Source: CAD feature listing. Evaluate the final solid. Frame: model axes, mm. A direction names the side the tool comes from. Coordinates: 2 decimals unless noted, no trailing zeros. Write each loop counter-clockwise with the first axis right and the second up, starting at its lowest first coordinate (ties: lowest second). Pieces come first, ordered by that corner, then holes. Notation, with made-up numbers: (-16.75, 61.25) - (15.25, 61.25) arc R14 cw to (15.25, 68.25) - close; hole circle Ø6 at (14, 13.25). An arc over 180 degrees is marked (long way). One line per question, with ' | ' between items. Start each with the question number.
Q1. Access query for faces 1 (the face through (216.99, 45.35, -92.85)), 2 (the face through (110, 25, -100)), 3 (the face through (171, 23, -91)), 4 (the face through (12.72, 11.89, -33.46)). Directions: +Z, -Z, +X, -X, +Y, -Y. A direction counts if a zero-diameter tool reaches every point of the face in a straight line with its end or side. Return the directions, or none.
Q2. Cut plane D-D, the plane z = -15. Return loops of the section in (x, y), plus the area to 3 significant figures.
Q3. Cut plane A-A, the plane y = 51.5. Give the number of separate pieces and of enclosed holes in the cut face, plus the area to 3 significant figures.
Q4. Cut plane C-C, the plane y = 12.5. Return loops of the section in (x, z).
Q5. Draft query along X for faces 5 (the face through (18, 5, -45)), 6 (the face through (108, 20, -51)), 7 (the face through (220, 9, -55)). Return one class per face: +X half, -X half, draft (parallel to the pull), parting line (faces both ways), or undercut.
Q6. Cut plane B-B, the plane x = 110. Return loops of the section in (y, z).
Q7. Line query: line 1 (X direction, y = 16, z = -44.5); line 2 (Z direction, x = 202, y = 8); line 3 (X direction, y = 11.25, z = -15). Output: solid intervals per line, ascending.
Q8. Contact query for flat-ended pins moving along their axis: P1, Ø4.5, axis at x = 43.5, z = -106, coming from the +Y side; P2, Ø10, axis at x = 111, z = -37, coming from the -Y side; P3, Ø18.5, axis at x = 107.5, z = -15.5, coming from the +Y side; P4, Ø25, axis at x = 72, y = 55, coming from the +Z side. Output: stop coordinate, or through.
```python
from build123d import *

# Parameters (mm, degrees)
SKETCH1_W           = 220
SKETCH1_H           = 110
BOSS_EXTRUDE1_DEPTH = 20
SKETCH2_R           = 12.49
SKETCH2_R_2         = 7.6
CUT_EXTRUDE1_DEPTH  = 15
SKETCH3_W           = 220
SKETCH3_H           = 20
BOSS_EXTRUDE2_DEPTH = 50
CHAMFER1_SIZE       = 1
FILLET1_R           = 1
FILLET2_R           = 10
SKETCH4_R           = 11.5
CUT_EXTRUDE2_DEPTH  = 5
SKETCH5_W           = 46.94076836
SKETCH5_H           = 60
SKETCH5_W_2         = 45
SKETCH5_H_2         = 90
CUT_EXTRUDE3_DEPTH  = 256.734237051
FILLET4_R           = 5
SKETCH6_R           = 3.2
CUT_EXTRUDE4_DEPTH  = 10


with BuildPart() as part:
    # Sketch1 → Boss-Extrude1 (new body)
    with BuildSketch(Plane(origin=(0, 0, 0), x_dir=(1, 0, 0), z_dir=(0, 1, 0))):
        with Locations((110, 55)):
            Rectangle(SKETCH1_W, SKETCH1_H)
    extrude(amount=BOSS_EXTRUDE1_DEPTH)

    # Sketch2 → Cut-Extrude1 (cut)
    with BuildSketch(Plane(origin=(0, 20, 0), x_dir=(1, 0, 0), z_dir=(0, 1, 0))):
        with Locations(Location((17.5, 45, 0), (0, 0, 270))):
            Circle(SKETCH2_R)
        with Locations(Location((202.5, 45, 0), (0, 0, 90))):
            Circle(SKETCH2_R)
        with Locations(Location((110, 15, 0), (0, 0, 270))):
            Circle(SKETCH2_R_2)
    extrude(amount=-CUT_EXTRUDE1_DEPTH, mode=Mode.SUBTRACT)

    # Sketch3 → Boss-Extrude2 (add)
    with BuildSketch(Plane(origin=(0, 20, 0), x_dir=(1, 0, 0), z_dir=(0, 1, 0))):
        with Locations((110, 100)):
            Rectangle(SKETCH3_W, SKETCH3_H)
    extrude(amount=BOSS_EXTRUDE2_DEPTH)

    # Chamfer1
    chamfer1_edges = [part.edges().sort_by_distance(p)[0] for p in [
        (17.5, 20, -57.49),
        (202.5, 20, -32.51),
    ]]
    chamfer(chamfer1_edges, length=CHAMFER1_SIZE)

    # Fillet1
    fillet1_edges = [part.edges().sort_by_distance(p)[0] for p in [
        (202.5, 19, -32.51),
        (17.5, 19, -57.49),
    ]]
    fillet(fillet1_edges, radius=FILLET1_R)

    # Fillet2
    fillet2_edges = [part.edges().sort_by_distance(p)[0] for p in [
        (220, 45, -90),
        (0, 45, -90),
        (0, 35, -110),
        (0, 10, 0),
        (220, 35, -110),
        (220, 10, 0),
    ]]
    fillet(fillet2_edges, radius=FILLET2_R - 0.0001)  # a hair under: the kernel refuses the full size

    # Sketch4 → Cut-Extrude2 (cut)
    with BuildSketch(Plane(origin=(0, 20, 0), x_dir=(1, 0, 0), z_dir=(0, 1, 0))):
        with Locations(Location((110, 15, 0), (0, 0, 270))):
            Circle(SKETCH4_R)
    extrude(amount=-CUT_EXTRUDE2_DEPTH, mode=Mode.SUBTRACT)

    # Sketch5 → Cut-Extrude3 (cut, through all)
    with BuildSketch(Plane(origin=(0, 0, -110), x_dir=(-1, 0, 0), z_dir=(0, 0, -1))):
        with Locations((-171.52961582, 55)):
            Rectangle(SKETCH5_W, SKETCH5_H)
        with Locations((-48.47038418, 55)):
            Rectangle(SKETCH5_W, SKETCH5_H)
        with Locations((-110, 70)):
            Rectangle(SKETCH5_W_2, SKETCH5_H_2)
    extrude(amount=-CUT_EXTRUDE3_DEPTH, mode=Mode.SUBTRACT)

    # Fillet4
    fillet4_edges = [part.edges().sort_by_distance(p)[0] for p in [
        (195, 47.5, -90),
        (148.05923164, 47.5, -90),
        (25, 47.5, -90),
        (71.94076836, 47.5, -90),
        (171.52961582, 25, -90),
        (48.47038418, 25, -90),
        (25, 70, -100),
        (25, 25, -100),
        (71.94076836, 25, -100),
        (71.94076836, 70, -100),
        (87.5, 70, -100),
        (87.5, 25, -100),
        (132.5, 25, -100),
        (132.5, 70, -100),
        (148.05923164, 70, -100),
        (148.05923164, 25, -100),
        (195, 25, -100),
    ]]
    fillet(fillet4_edges, radius=FILLET4_R - 0.0001)  # a hair under: the kernel refuses the full size

    # Sketch6 → Cut-Extrude4 (cut)
    with BuildSketch(Plane(origin=(0, 0, -110), x_dir=(-1, 0, 0), z_dir=(0, 0, -1))):
        with Locations((-110, 12.5)):
            Circle(SKETCH6_R)
    extrude(amount=-CUT_EXTRUDE4_DEPTH, mode=Mode.SUBTRACT)


solid = part.part
```
Reply:
1) face 1: +Z, +X, +Y | face 2: +Z, -Z, +Y | face 3: +Z, +Y | face 4: +Y
2) outline: (0, 0) - (220, 0) - (220, 20) - (121.5, 20) - (121.5, 15) - (117.6, 15) - (117.6, 5) - (102.4, 5) - (102.4, 15) - (98.5, 15) - (98.5, 20) - (0, 20) - close | area: 4,130 mm^2
3) separate pieces: 4 | enclosed holes: 0 | area: 1,520 mm^2
4) outline: (0, -100) arc R10 ccw to (10, -110) - (106.8, -110) - (106.8, -100) - (113.2, -100) - (113.2, -110) - (210, -110) arc R10 ccw to (220, -100) - (220, -10) arc R10 ccw to (210, 0) - (10, 0) arc R10 ccw to (0, -10) - close; hole circle Ø24.98 at (17.5, -45); hole circle Ø15.2 at (110, -15); hole circle Ø24.98 at (202.5, -45)
5) face 5: undercut | face 6: draft | face 7: +X half
6) outline: (0, -110) - (9.3, -110) - (9.3, -100) - (15.7, -100) - (15.7, -110) - (25, -110) - (25, -90) - (20, -90) - (20, -26.5) - (15, -26.5) - (15, -22.6) - (5, -22.6) - (5, -7.4) - (15, -7.4) - (15, -3.5) - (20, -3.5) - (20, 0) - (0, 0) - close
7) line 1: x = 0 to 5.02, 29.98 to 190.02, 214.98 to 220 | line 2: z = -110 to -57.48, -32.52 to 0 | line 3: x = 0 to 102.4, 117.6 to 220
8) P1: stops at y = 25 | P2: stops at y = 0 | P3: stops at y = 20 | P4: stops at z = -90
